```python
from build123d import *

# Parameters (mm, degrees)
SKETCH1_W           = 180
SKETCH1_H           = 180
BOSS_EXTRUDE1_DEPTH = 5
CUT_EXTRUDE1_DEPTH  = 128.377392029
SKETCH4_R           = 3.1
CUT_EXTRUDE2_DEPTH  = 128.377392029
SKETCH5_R           = 3.1
CUT_EXTRUDE3_DEPTH  = 128.377392029
SKETCH6_R           = 2.1
CUT_EXTRUDE4_DEPTH  = 128.377392029


with BuildPart() as part:
    # Sketch1 → Boss-Extrude1 (new body)
    with BuildSketch(Plane.XY):
        Rectangle(SKETCH1_W, SKETCH1_H)
    extrude(amount=BOSS_EXTRUDE1_DEPTH)

    # Sketch3 → Cut-Extrude1 (cut, through all)
    with BuildSketch(Plane(origin=(0, 0, 0), x_dir=(-1, 0, 0), z_dir=(0, 0, -1))):
        with BuildLine():
            Line((-34.154155691, -13.446054827), (23.801393887, 2.083087879))
            ThreePointArc((23.801393887, 2.083087879), (48.296291314, -12.059047745), (34.154155691, -36.553945173))
            Line((34.154155691, -36.553945173), (-23.801393887, -52.083087879))
            ThreePointArc((-23.801393887, -52.083087879), (-48.296291314, -37.940952255), (-34.154155691, -13.446054827))
        make_face()
    extrude(amount=-CUT_EXTRUDE1_DEPTH, mode=Mode.SUBTRACT)

    # Sketch4 → Cut-Extrude2 (cut, through all)
    with BuildSketch(Plane.XY.offset(5)):
        with Locations((-65, 80)):
            Circle(SKETCH4_R)
        with Locations((-65, 40)):
            Circle(SKETCH4_R)
        with Locations((-65, 0)):
            Circle(SKETCH4_R)
        with Locations((-65, -40)):
            Circle(SKETCH4_R)
    extrude(amount=-CUT_EXTRUDE2_DEPTH, mode=Mode.SUBTRACT)

    # Sketch5 → Cut-Extrude3 (cut, through all)
    with BuildSketch(Plane(origin=(0, 0, 0), x_dir=(-1, 0, 0), z_dir=(0, 0, -1))):
        with Locations((-74.600409008, 80)):
            Circle(SKETCH5_R)
        with Locations((-74.600409008, 40)):
            Circle(SKETCH5_R)
        with Locations((-74.600409008, 0)):
            Circle(SKETCH5_R)
        with Locations((-74.600409008, -40)):
            Circle(SKETCH5_R)
    extrude(amount=-CUT_EXTRUDE3_DEPTH, mode=Mode.SUBTRACT)

    # Sketch6 → Cut-Extrude4 (cut, through all)
    with BuildSketch(Plane(origin=(0, 0, 0), x_dir=(-1, 0, 0), z_dir=(0, 0, -1))):
        with Locations((-7.764571353, 3.977774789)):
            Circle(SKETCH6_R)
        with Locations(Location((7.764571353, -53.977774789, 0), (0, 0, 180))):
            Circle(SKETCH6_R)
        with Locations(Location((46.401604405, -43.625012985, 0), (0, 0, 180))):
            Circle(SKETCH6_R)
        with Locations((30.872461698, 14.330536593)):
            Circle(SKETCH6_R)
        with Locations((-30.872461698, -64.330536593)):
            Circle(SKETCH6_R)
        with Locations(Location((-46.401604405, -6.374987015, 0), (0, 0, 180))):
            Circle(SKETCH6_R)
    extrude(amount=-CUT_EXTRUDE4_DEPTH, mode=Mode.SUBTRACT)


solid = part.part
```
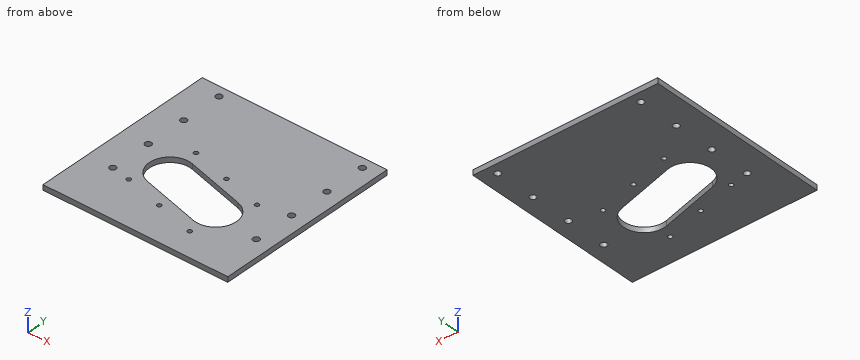
For this review, take the finished solid that the model builds, in its own axes (mm). Round coordinates to 2 decimals unless told otherwise and drop trailing zeros. Write each loop counter-clockwise with the first axis right and the second up, starting at its lowest first coordinate (ties: lowest second). Pieces come first, ordered by that corner, then holes. Notation, with made-up numbers: (82, 56.5) - (134, 56.5) arc R19 ccw to (134, 64.5) - close; hole circle Ø5 at (82, -16.75). An arc over 180 degrees is marked (long way). Answer as CSV lines item,"result". Start each with the question number.
(1) Add section A-A, the plane y = 80. State the section outline as (x, z) points.
(2) For pin 1 (5.5 mm diameter, centred on x = 74.6, y = 80, fed in from +Z), flat-tipped, find the tip position at first contact; note if it passes through.
(3) Add section D-D, the plane y = -24. State the section outline as (x, z) points, plus the area to 3 significant figures.
(4) For line 1 (Y direction, x = -65, z = 3.9); line 2 (Y direction, x = -14, z = 2.85); line 3 (Y direction, x = -7.5, z = 3.2), list the stretches that pass through material, from the lowest coordinate up.
(5) Add section B-B, the plane x = 37.5. State the section outline as (y, z) points.
(6) Add section C-C, the plane x = -65. State the section outline as (y, z) points, plus the area to 3 significant figures.
From the geometry:
1,outline,"(-90, 0) - (-68.1, 0) - (-68.1, 5) - (-90, 5) - close; (-61.9, 0) - (71.5, 0) - (71.5, 5) - (-61.9, 5) - close; (77.7, 0) - (90, 0) - (90, 5) - (77.7, 5) - close"
2,pin 1,"passes through"
3,outline,"(-90, 0) - (-47.8, 0) - (-47.8, 5) - (-90, 5) - close; (46.96, 0) - (90, 0) - (90, 5) - (46.96, 5) - close"
3,area,"426 mm²"
4,line 1,"y = -90 to -43.1, -36.9 to -3.1, 3.1 to 36.9, 43.1 to 76.9, 83.1 to 90"
4,line 2,"y = -90 to -41.95, -0.54 to 90"
4,line 3,"y = -90 to -56.06, -51.89 to -43.7, -2.28 to 90"
5,outline,"(-90, 0) - (-50.86, 0) - (-50.86, 5) - (-90, 5) - close; (-14.67, 0) - (90, 0) - (90, 5) - (-14.67, 5) - close"
6,outline,"(-90, 0) - (-43.1, 0) - (-43.1, 5) - (-90, 5) - close; (-36.9, 0) - (-3.1, 0) - (-3.1, 5) - (-36.9, 5) - close; (3.1, 0) - (36.9, 0) - (36.9, 5) - (3.1, 5) - close; (43.1, 0) - (76.9, 0) - (76.9, 5) - (43.1, 5) - close; (83.1, 0) - (90, 0) - (90, 5) - (83.1, 5) - close"
6,area,"776 mm²"
